The figure shows three views and two pictorial views of one solid part (mm, origin at its lowest corner). Answer the questions. A direction names the side the tool comes from. Round coordinates to 2 decimals unless told otherwise and drop trailing zeros. Write each loop counter-clockwise with the first axis right and the second up, starting at its lowest first coordinate (ties: lowest second). Pieces come first, ordered by that corner, then holes. Notation, with made-up numbers: (11.5, 56) -> (44.5, 56) arc R20 ccw to (44.5, 90) -> close; hole circle Ø9 at (-30.75, -20.5). An arc over 180 degrees is marked (long way). One line per item, written item: value.
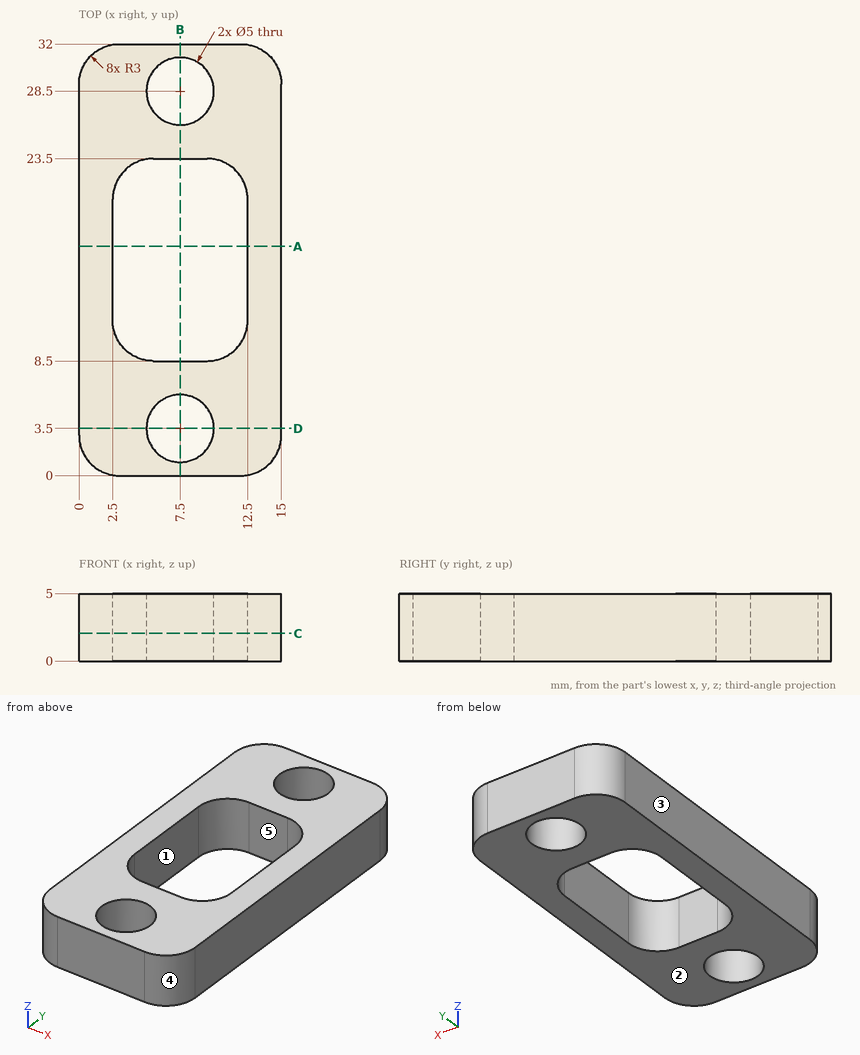
(1) Find section C-C on z = 2.05. Give the vertices of the cut face in (x, y).
Reported:
outline: (0, 3) arc R3 ccw to (3, 0) -> (12, 0) arc R3 ccw to (15, 3) -> (15, 29) arc R3 ccw to (12, 32) -> (3, 32) arc R3 ccw to (0, 29) -> close; hole (2.5, 11.5) arc R3 ccw to (5.5, 8.5) -> (9.5, 8.5) arc R3 ccw to (12.5, 11.5) -> (12.5, 20.5) arc R3 ccw to (9.5, 23.5) -> (5.5, 23.5) arc R3 ccw to (2.5, 20.5) -> close; hole circle Ø5 at (7.5, 3.5); hole circle Ø5 at (7.5, 28.5)
(2) Find section A-A on y = 17. Give the vertices of the cut face in (x, z), plus the area to 3 significant figures.
Reported:
outline: (0, 0) -> (2.5, 0) -> (2.5, 5) -> (0, 5) -> close; (12.5, 0) -> (15, 0) -> (15, 5) -> (12.5, 5) -> close
area: 25.0 mm2
(3) A tool of negligible diameter and unlimited length cuts with its end or side. For the marked faces 1 and 2, from which of +Z, -Z, +X, -X, +Y, -Y can it reach the whole face along a straight path? Write none if from no direction.
Reported:
face 1: +Z, -Z
face 2: -Z, +X, -X, +Y, -Y
(4) For a pull along X with two mould halves and no side action, classify the marked faces 3, 4 and 5 as pulls with the +X half, pulls with the -X half, needs draft (parallel to the pull), parting line crosses it, or undercut.
Reported:
face 3: pulls with the -X half
face 4: pulls with the +X half
face 5: undercut
(5) Consider probe 1 along Y at (x, z) = (7.5, 1.25); probe 2 along X at (y, z) = (16, 1.95); probe 3 along Y at (x, z) = (9.5, 2.4). Determine where each line is inside the solid, lowest interval first.
Reported:
probe 1: y = 0 to 1, 6 to 8.5, 23.5 to 26, 31 to 32
probe 2: x = 0 to 2.5, 12.5 to 15
probe 3: y = 0 to 2, 5 to 8.5, 23.5 to 27, 30 to 32
(6) Find section D-D on y = 3.5. Give the vertices of the cut face in (x, z), plus the area to 3 significant figures.
Reported:
outline: (0, 0) -> (5, 0) -> (5, 5) -> (0, 5) -> close; (10, 0) -> (15, 0) -> (15, 5) -> (10, 5) -> close
area: 50.0 mm2
(7) Find section B-B on x = 7.5. Give the vertices of the cut face in (y, z).
Reported:
outline: (0, 0) -> (1, 0) -> (1, 5) -> (0, 5) -> close; (6, 0) -> (8.5, 0) -> (8.5, 5) -> (6, 5) -> close; (23.5, 0) -> (26, 0) -> (26, 5) -> (23.5, 5) -> close; (31, 0) -> (32, 0) -> (32, 5) -> (31, 5) -> close
(8) A flat-ended cylindrical pin translates along its axis: pin 1 Ø4.5 at (x, y) = (7.5, 28.5) entering from -Z. Find the tip coordinate at first contact, or state that the pin passes through.
Reported:
pin 1: passes through
